Could you check a few things on this drawing? It's one solid part, dimensions in mm from its lowest x, y, z. Coordinates: 2 decimals unless noted, no trailing zeros. Write each loop counter-clockwise with the first axis right and the second up, starting at its lowest first coordinate (ties: lowest second). Pieces come first, ordered by that corner, then holes.
Item 1: I want a section at A-A (x = 116.5). Please give me the cut outline in (y, z).
Item 2: I'm going to push flat-ended pins straight in: P1, Ø1, axis at x = 53.5, z = 0.5, coming from the +Y side; P2, Ø1, axis at x = 55.5, z = 2, coming from the +Y side; P3, Ø5, axis at x = 98.5, y = 4.5, coming from the -Z side. Where does each tip first touch, or does it pass through?
Item 3: I want a section at D-D (x = 142). Please give me the cut outline in (y, z).
Item 4: Please list where these lines run through material, in increasing order: line 1 (Y direction, x = 99, z = 0.3) (1 decimal); line 2 (Y direction, x = 157, z = 1.1); line 3 (X direction, y = 4, z = 0.8) (1 decimal).
Item 5: I want a section at B-B (y = 48). Please give me the cut outline in (x, z) (1 decimal).
Item 6: I want a section at C-C (z = 0.35). Count the separate pieces of the cut face and the enclosed holes in it.
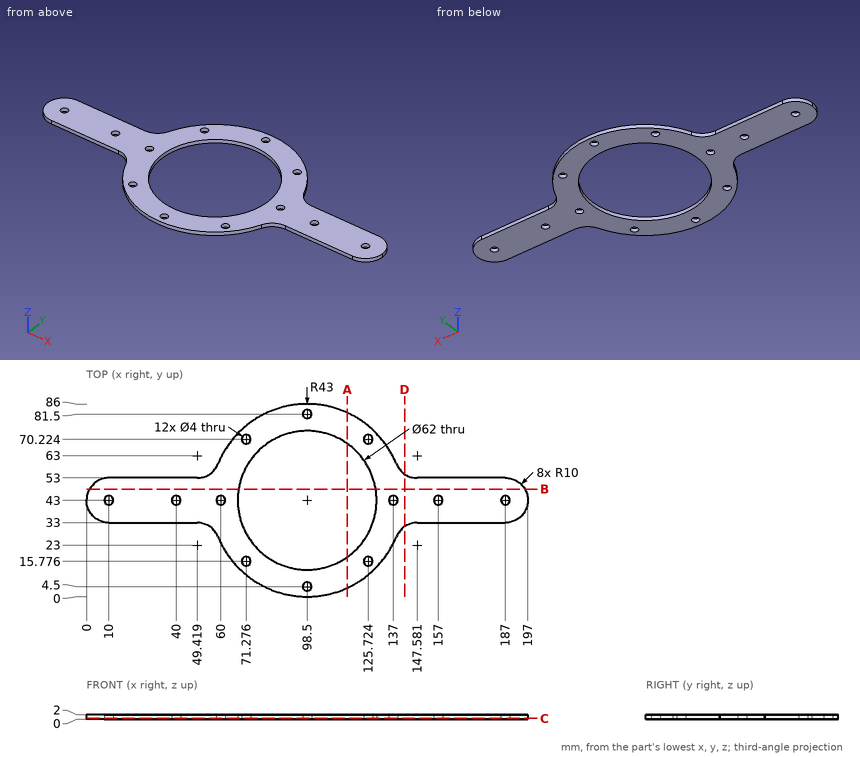
Answer:
1. outline: (3.95, 0) - (17.76, 0) - (17.76, 2) - (3.95, 2) - close; (68.24, 0) - (82.05, 0) - (82.05, 2) - (68.24, 2) - close
2. P1: stops at y = 54.11
2. P2: stops at y = 55.47
2. P3: stops at z = 0
3. outline: (31.3, 0) - (54.7, 0) - (54.7, 2) - (31.3, 2) - close
4. line 1: y = 0 to 2.6, 6.4 to 12, 74 to 79.6, 83.4 to 86
4. line 2: y = 33 to 41, 45 to 53
4. line 3: x = 80.4 to 96.6, 100.4 to 116.6
5. outline: (1.3, 0) - (67.9, 0) - (67.9, 2) - (1.3, 2) - close; (129.1, 0) - (195.7, 0) - (195.7, 2) - (129.1, 2) - close
6. separate pieces: 1
6. enclosed holes: 13
